Geometry check sheet. Reference: the model listing, model coordinates, mm. Face numbers are marked on the shaded views. A direction names the side the tool comes from. Round coordinates to 2 decimals unless told otherwise and drop trailing zeros. Order: outer loops, then holes, each group sorted by start corner. A loop starts at its lowest first (then second) coordinate and runs counter-clockwise, first axis right, second up. Notation, with made-up numbers: (-38.5, 49) - (-8.5, 49) arc R30 ccw to (-8.5, 77) - close; hole circle Ø5 at (-17.75, 63.5). An arc over 180 degrees is marked (long way). One line per question, with ' | ' between items. Start each with the question number.
Q1. Sectioned sample at A-A, the plane z = 0. Enter the section's corners in (x, y).
Q2. Mould release check, pull along Z, two halves, no side actions. Record for the marked faces 1 and 2: +Z half, -Z half, draft (parallel to the pull), parting line (faces both ways), or undercut.
Q3. Tool access check on the marked faces 3, 4 and 5. Record the directions out of +Z, -Z, +X, -X, +Y, -Y that give a thin tool (end or side, any length) a straight path to the whole face; none if there is none.
Q4. Gauge pin test, flat end, axial feed: P1, Ø1.5, axis at y = 2, z = -5, coming from the -X side. Record the tip position at first contact, or that the pin passes through.
Q5. Sectioned sample at D-D, the plane y = 0.55. Enter the section's corners in (x, z), then the cut area to 3 significant figures.
Q6. Sectioned sample at B-B, the plane x = 0. Enter the section's corners in (y, z).
Q7. Material ranges on line 1 along Z through (x, y) = (0, 3.8); line 2 along Y through (x, z) = (-3.75, -2.25); line 3 along Y through (x, z) = (2, -5.75), recorded low to high.
Q8. Sectioned sample at C-C, the plane y = 2.8. Enter the section's corners in (x, z), then the cut area to 3 significant figures.
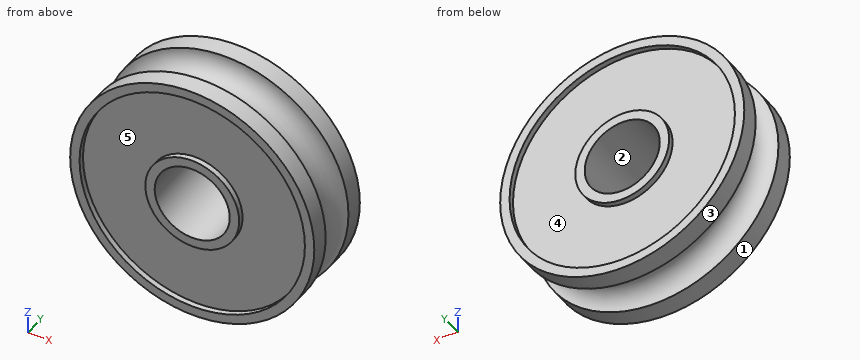
Autodesk Inventor part; units mm, degrees
ref_plane "РабПлоскость1" through (0, 2, 0) normal (0, 1, 0) x (1, 0, 0)
ref_plane "РабПлоскость2" through (0, 0, 0) normal (0, 0, 1) x (1, 0, 0)
ref_plane "YZ Plane" through (0, 0, 0) normal (1, 0, 0) x (0, 1, 0)
sketch "Эскиз1" plane through (0, 0, 0) normal (0, 1, 0) x (-1, 0, 0)
  circle A0 centre (0, 0) radius 2
  circle A1 centre (0, 0) radius 6.5
  dimension "d1" = 4
  dimension "d2" = 13
extrude "Выдавливание1" add sketch "Эскиз1" along normal blind 4
sketch "Эскиз2" plane through (0, 4, 0) normal (0, 1, 0) x (1, 0, 0)
  circle A0 centre (0, 0) radius 2
  circle A1 centre (0, 0) radius 2.5
  circle A2 centre (0, 0) radius 6
  dimension "d5" = 5
  dimension "d6" = 12
extrude "Выдавливание2" cut sketch "Эскиз2" against normal blind 0.3 contours A2
sketch "Эскиз3" plane through (0, 0, 0) normal (0, -1, 0) x (1, 0, 0)
  circle A0 centre (0, 0) radius 2.5
  circle A1 centre (0, 0) radius 6
  dimension "d9" = 5
  dimension "d10" = 12
extrude "Выдавливание3" cut sketch "Эскиз3" against normal blind 0.3
ref_plane "РабПлоскость1" through (0, 2, 0) normal (0, 1, 0) x (1, 0, 0)
sketch "Эскиз4" plane through (0, 2, 0) normal (0, 1, 0) x (1, 0, 0)
  circle A0 centre (0, 0) radius 6.5
  dimension "d13" = 13
ref_plane "РабПлоскость2" through (0, 0, 0) normal (0, 0, 1) x (1, 0, 0)
sketch "Эскиз6" plane through (0, 0, 0) normal (0, 0, 1) x (1, 0, 0)
  line L0 (-6.5, 0) -> (-6.5, 4)
  circle A0 centre (-6.5, 2) radius 1
  line L1 (0, -0.8) -> (0, 4.8)
  point P0 (0, 0)
  dimension "d15" = 2
revolve "Вращение1" cut sketch "Эскиз6" angle 360 about axis through (0, -10, 0) along (0, 1, 0)
properties part number "U-подшипник"
Determined:
1) outline: (-6.5, 0) - (-6, 0) - (-6, 0.3) - (-2.5, 0.3) - (-2.5, 0) - (-2, 0) - (-2, 4) - (-2.5, 4) - (-2.5, 3.7) - (-6, 3.7) - (-6, 4) - (-6.5, 4) - (-6.5, 3) arc R1 cw to (-6.5, 1) - close; (2, 0) - (2.5, 0) - (2.5, 0.3) - (6, 0.3) - (6, 0) - (6.5, 0) - (6.5, 1) arc R1 cw to (6.5, 3) - (6.5, 4) - (6, 4) - (6, 3.7) - (2.5, 3.7) - (2.5, 4) - (2, 4) - close
2) face 1: parting line | face 2: undercut
3) face 3: +Y, -Y | face 4: +Y | face 5: -Y
4) P1: stops at x = -3.49
5) outline: circle Ø13 at (0, 0); hole circle Ø4 at (0, 0) | area: 120 mm2
6) outline: (0, -6.5) - (1, -6.5) arc R1 cw to (3, -6.5) - (4, -6.5) - (4, -6) - (3.7, -6) - (3.7, -2.5) - (4, -2.5) - (4, -2) - (0, -2) - (0, -2.5) - (0.3, -2.5) - (0.3, -6) - (0, -6) - close; (0, 2) - (4, 2) - (4, 2.5) - (3.7, 2.5) - (3.7, 6) - (4, 6) - (4, 6.5) - (3, 6.5) arc R1 cw to (1, 6.5) - (0, 6.5) - (0, 6) - (0.3, 6) - (0.3, 2.5) - (0, 2.5) - close
7) line 1: z = -6.5 to -6, -2.5 to -2, 2 to 2.5, 6 to 6.5 | line 2: y = 0.3 to 3.7 | line 3: y = 0 to 1.09, 2.91 to 4
8) outline: circle Ø11.8 at (0, 0); hole circle Ø4 at (0, 0) | area: 96.8 mm2
